Check sheet for the modelled part. Datum: model origin and axes. Units: mm. Face numbers are marked on the shaded views. A direction names the side the tool comes from. Coordinates: 2 decimals unless noted, no trailing zeros. Loops run counter-clockwise (first coordinate to the right, second up) from the corner with the lowest first, then second, coordinate; pieces in that order, holes last.
Autodesk Inventor part; units mm, degrees
ref_plane "YZ Plane" through (0, 0, 0) normal (1, 0, 0) x (0, 1, 0)
ref_plane "XZ Plane" through (0, 0, 0) normal (0, 1, 0) x (-1, 0, 0)
ref_plane "XY Plane" through (0, 0, 0) normal (0, 0, 1) x (1, 0, 0)
sketch "Sketch1" plane through (0, 0, 0) normal (1, 0, 0) x (0, 1, 0)
  line L0 (0, 0) -> (15, 0)
  line L1 (15, 0) -> (15, -40)
  line L2 (15, -40) -> (0, -40)
  line L3 (0, -40) -> (0, 0)
  dimension "d0" = 40
  dimension "d1" = 15
extrude "Extrusion1" add sketch "Sketch1" along normal mid plane 25
sketch "Sketch2" plane through (12.5, 0, 0) normal (1, 0, 0) x (0, 0, -1)
  line L0 (-5, 16.2216) -> (25, 16.2216)
  line L1 (25, 16.2216) -> (25, 7.5)
  line L2 (25, 7.5) -> (-5, 7.5)
  line L3 (-5, 7.5) -> (-5, 16.2216)
  line L4 (40, 0) -> (40, 15)
  line L5 (0, 0) -> (40, 0)
  dimension "d4" = 15
  dimension "d5" = 30
  dimension "d6" = 7.5
extrude "Extrusion2" cut sketch "Sketch2" against normal through all
sketch "Sketch3" plane through (-12.5, 15, -40) normal (0, 1, 0) x (1, 0, 0)
  point P0 (12.5, -40)
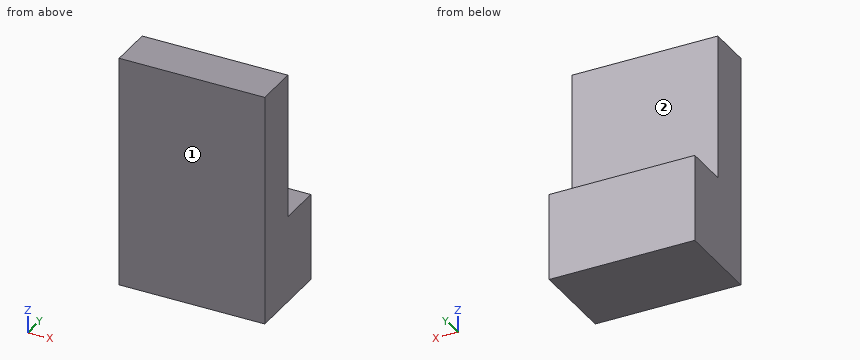
1) Section check A-A on x = 8.5. Enter the section's corners in (y, z), plus the area to 4 significant figures.
Answer sheet:
outline: (0, -40) - (15, -40) - (15, -25) - (7.5, -25) - (7.5, 0) - (0, 0) - close
area: 412.5 mm2
2) Section check C-C on z = -24. Enter the section's corners in (x, y), plus the area to 4 significant figures.
Answer sheet:
outline: (-12.5, 0) - (12.5, 0) - (12.5, 7.5) - (-12.5, 7.5) - close
area: 187.5 mm2
3) Set-up check for the marked faces 1 and 2: record each of +Z, -Z, +X, -X, +Y, -Y from which the full face is reachable in a straight line by a thin tool's end or side.
Answer sheet:
face 1: +Z, -Z, +X, -X, -Y
face 2: +Z, +X, -X, +Y
4) Depth check by flat-ended pin: pin 1 (12 mm diameter, centred on x = 7, z = -13.5, fed in from +Y). Enter the tip coordinate at first touch or a pass-through.
Answer sheet:
pin 1: stops at y = 7.5
5) Scan lines: line 1 (Y direction, x = 10.75, z = -13); line 2 (Z direction, x = -1.25, y = 8.75). Record each from-to range of solid material in increasing order.
Answer sheet:
line 1: y = 0 to 7.5
line 2: z = -40 to -25
6) Section check B-B on y = 8.25. Enter the section's corners in (x, z), plus the area to 3 significant figures.
Answer sheet:
outline: (-12.5, -40) - (12.5, -40) - (12.5, -25) - (-12.5, -25) - close
area: 375 mm2
